Print and shaded views of the part. All mm, measured from the part's lowest x, y and z. A direction names the side the tool comes from. Give positions to 0.01 mm unless a question says otherwise; leave off trailing zeros. Loops run counter-clockwise (first coordinate to the right, second up) from the corner with the lowest first, then second, coordinate; pieces in that order, holes last. Notation, with made-up numbers: (62.5, 81) - (103.5, 81) arc R25 cw to (103.5, 100) - close; hole circle Ø6 at (13, 50). An arc over 180 degrees is marked (long way). Return JSON: item names as keys, results as strings.
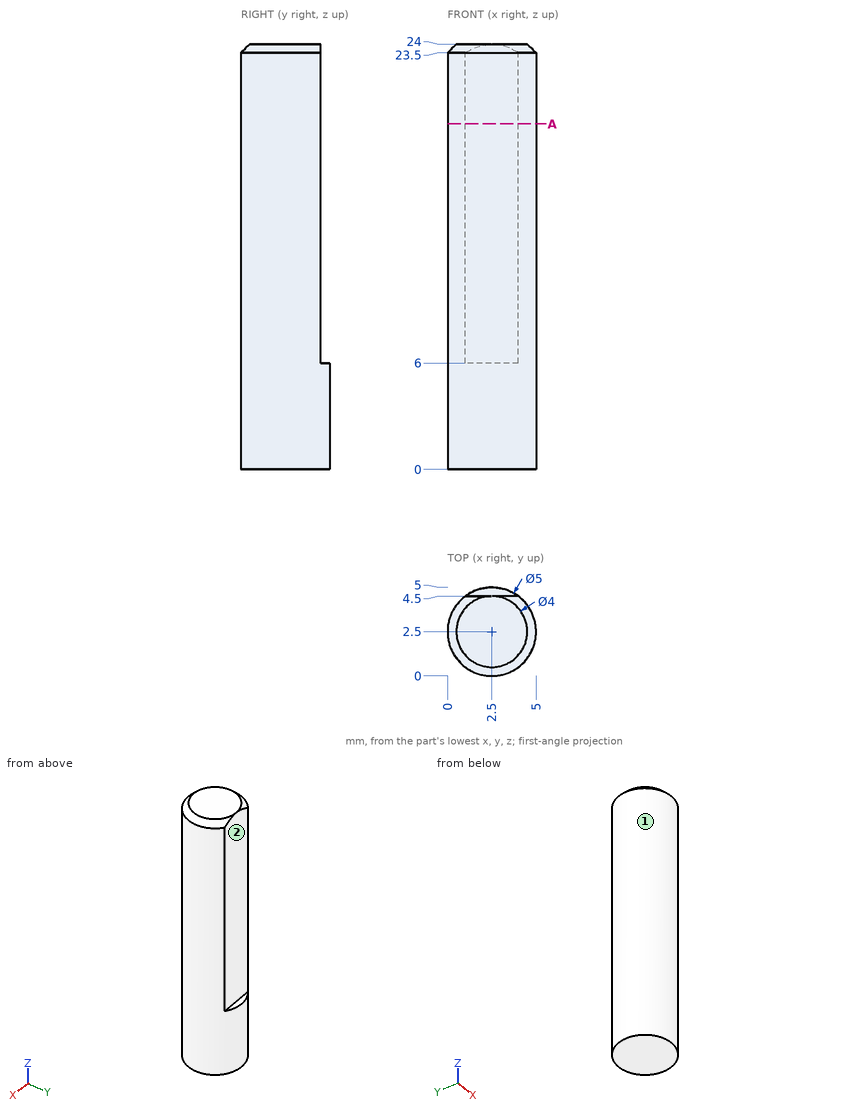
1. Drop flat-ended pins along their axis: P1, Ø2, axis at y = 0.5, z = 5.5, coming from the +X side; P2, Ø1, axis at y = 1.5, z = 11, coming from the +X side; P3, Ø1.5, axis at x = 2, z = 13, coming from the +Y side. Give the stop position or say it passes through.
Values follow:
{"P1": "stops at x = 4.79", "P2": "stops at x = 4.95", "P3": "stops at y = 4.5"}
2. Cut at A-A, the plane z = 19.5. Write the cut outline in (x, y).
Values follow:
{"outline": "(1, 4.5) arc R2.5 ccw (long way) to (4, 4.5) - close"}
3. Which spindle directions (+Z, -Z, +X, -X, +Y, -Y) get a long thin tool onto all of the face, cutting with end or side? Do the marked faces 1 and 2. Say none if no direction does.
Values follow:
{"face 1": "+Z, -Z", "face 2": "+Z, +X, -X, +Y"}
4. Drill centre lines: probe 1 along Y at (x, z) = (2.65, 4.5); probe 2 along X at (y, z) = (0.5, 7.75); probe 3 along Y at (x, z) = (1.3, 9). Where is each one in solid material? Low to high.
Values follow:
{"probe 1": "y = 0 to 5", "probe 2": "x = 1 to 4", "probe 3": "y = 0.31 to 4.5"}
